Work out the finished part from the listing and answer in its coordinate system (mm). A direction names the side the tool comes from. Round coordinates to 2 decimals unless told otherwise and drop trailing zeros. Order: outer loops, then holes, each group sorted by start corner. A loop starts at its lowest first (then second) coordinate and runs counter-clockwise, first axis right, second up. Notation, with made-up numbers: (-19, 18.25) - (22, 18.25) arc R23 cw to (22, 55.25) - close; hole circle Ø8 at (-5, -4). An arc over 180 degrees is marked (long way). Use one line per item in the form item = value. Start each with the question number.
Q1. The part is cut by section A-A on x = 2. Determine the outline of the cut face in (y, z), plus the area to 3 significant figures.
Q2. Which of the six approach directions +Z, -Z, +X, -X, +Y, -Y give full straight-line access (tool end or side, diameter ignored) to faces 5 (the flat face through (6, 74, -7)), 6 (the cylindrical face through (7.5, 36.98, 0.16)), 7 (the flat face through (1.83, 36.98, -3.24)), 8 (the flat face through (6, 2, 7)), 9 (the flat face through (5, 3, 7))?
Q3. Given P1, Ø4, axis at x = 4.5, y = 57, coming from the +Z side; P2, Ø2.5, axis at y = 1.5, z = 5.9, coming from the +X side; P3, Ø1.5, axis at y = 22.5, z = 0, coming from the -X side; P4, Ø1.3, axis at y = 73.5, z = 5.9, coming from the -X side, each flat-ended and moving along its own axis, determine where each tip first touches the part or whether it passes through.
Q4. For a pull along Z with two mould halves and no side action, classify faces 1 (the flat face through (0, 37, 6)), 2 (the flat face through (3.72, 37, 0)), 3 (the flat face through (3, 73, 7.5)), 4 (the flat face through (3, 1, -7.5)) as +Z half, -Z half, draft (parallel to the pull), parting line (faces both ways), or undercut.
Q5. The part is cut by section B-B on y = 1.5. Determine the outline of the cut face in (x, z), plus the area to 3 significant figures.
Q6. The part is cut by section C-C on y = 57. Determine the outline of the cut face in (x, z).
Q7. Find the intervals of material crossed by line 1 (Y direction, x = 3.25, z = 5.75); line 2 (Z direction, x = 3.95, y = 73.5); line 3 (Y direction, x = 4.25, z = 7), in increasing order. Write a range as [from, to].
Q8. The part is cut by section D-D on x = 5. Determine the outline of the cut face in (y, z), plus the area to 3 significant figures.
from build123d import *

# Parameters (mm, degrees)
MAIN_BODY_DEPTH                = 75
SKETCH2_W                      = 3.204513997
SKETCH2_H                      = 3
BACK_SCREW_HOLES_SUPPORT_DEPTH = 6
SKETCH3_R                      = 1.05
BACK_SCREW_HOLES_DEPTH         = 76.746287038


with BuildPart() as part:
    # Sketch1 → Main Body (new body)
    with BuildSketch(Plane(origin=(0, 0, 0), x_dir=(1, 0, 0), z_dir=(0, 1, 0))):
        with BuildLine():
            Line((0, 7.5), (0, 4.295486003))
            Line((0, 4.295486003), (3.72, 2.147743001))
            Line((3.72, 2.147743001), (3.72, -2.147743001))
            Line((3.72, -2.147743001), (0, -4.295486003))
            Line((0, -4.295486003), (0, -7.5))
            ThreePointArc((0, -7.5), (7.5, 0), (0, 7.5))
        make_face()
    extrude(amount=MAIN_BODY_DEPTH)

    # Sketch2 → Back Screw Holes Support (add)
    with BuildSketch(Plane.ZY):
        with Locations((-5.897743002, 1.5)):
            Rectangle(SKETCH2_W, SKETCH2_H)
        with Locations((-5.897743002, 73.5)):
            Rectangle(SKETCH2_W, SKETCH2_H)
    back_screw_holes_support = extrude(amount=-BACK_SCREW_HOLES_SUPPORT_DEPTH)

    # Sketch3 → Back Screw Holes (cut, through all)
    with BuildSketch(Plane.ZY):
        with Locations((-5.897743001, 73.5)):
            Circle(SKETCH3_R)
        with Locations((-5.897743001, 1.5)):
            Circle(SKETCH3_R)
    back_screw_holes = extrude(amount=-BACK_SCREW_HOLES_DEPTH, mode=Mode.SUBTRACT)

    # Front Screw Holes and Support: Back Screw Holes Support, Back Screw Holes across plane
    add(back_screw_holes_support.mirror(Plane.XY))
    add(back_screw_holes.mirror(Plane.XY), mode=Mode.SUBTRACT)


solid = part.part
Found:
q1.outline = (0, -7.5) - (3, -7.5) - (3, -7.23) - (72, -7.23) - (72, -7.5) - (75, -7.5) - (75, -3.14) - (0, -3.14) - close; (0, 3.14) - (75, 3.14) - (75, 7.5) - (72, 7.5) - (72, 7.23) - (3, 7.23) - (3, 7.5) - (0, 7.5) - close; hole circle Ø2.1 at (1.5, -5.9); hole circle Ø2.1 at (1.5, 5.9); hole circle Ø2.1 at (73.5, -5.9); hole circle Ø2.1 at (73.5, 5.9)
q1.area = 603 mm²
q2.face_5 = -Z, +X, +Y, -Y
q2.face_6 = +X
q2.face_7 = -X, +Y, -Y
q2.face_8 = +Z, +X, +Y, -Y
q2.face_9 = +Z, +X
q3.P1 = 7.07
q3.P2 = 6
q3.P3 = 3.72
q3.P4 = through
q4.face_1 = draft
q4.face_2 = undercut
q4.face_3 = +Z half
q4.face_4 = -Z half
q5.outline = (0, -7.5) - (6, -7.5) - (6, -6.95) - (0, -6.95) - close; (0, -4.85) - (6, -4.85) - (6, -4.5) arc R7.5 ccw to (6, 4.5) - (6, 4.85) - (0, 4.85) - (0, 4.3) - (3.72, 2.15) - (3.72, -2.15) - (0, -4.3) - close; (0, 6.95) - (6, 6.95) - (6, 7.5) - (0, 7.5) - close
q5.area = 50.0 mm²
q6.outline = (0, -7.5) arc R7.5 ccw to (0, 7.5) - (0, 4.3) - (3.72, 2.15) - (3.72, -2.15) - (0, -4.3) - close
q7.line_1 = [0, 0.46], [2.54, 72.46], [74.54, 75]
q7.line_2 = [-7.5, -6.95], [-4.85, 4.85], [6.95, 7.5]
q7.line_3 = [0, 3], [72, 75]
q8.outline = (0, -7.5) - (3, -7.5) - (3, -5.59) - (72, -5.59) - (72, -7.5) - (75, -7.5) - (75, 7.5) - (72, 7.5) - (72, 5.59) - (3, 5.59) - (3, 7.5) - (0, 7.5) - close; hole circle Ø2.1 at (1.5, -5.9); hole circle Ø2.1 at (1.5, 5.9); hole circle Ø2.1 at (73.5, -5.9); hole circle Ø2.1 at (73.5, 5.9)
q8.area = 848 mm²
